Geometry: see drawing. Coordinates: mm, zero at the bounding-box minimum. A direction names the side the tool comes from. Give positions to 0.01 mm unless a question says otherwise; leave off trailing zeros. Write each loop counter-clockwise with the first axis right and the second up, starting at its lowest first coordinate (ties: lowest second). Pieces come first, ordered by that corner, then holes.
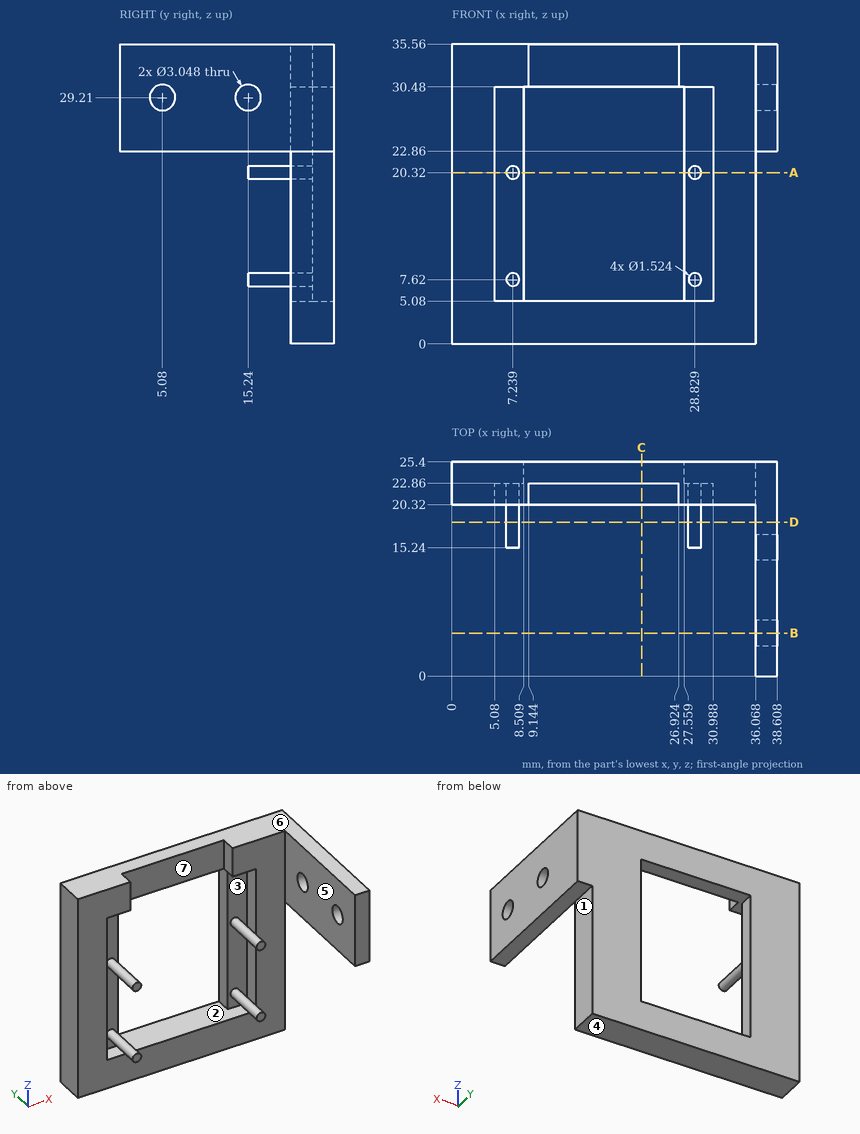
1. Pull-direction query (Z, two-part tool) for the marked faces 1, 2, 3 and 4; classes: pulls with the +Z half, pulls with the -Z half, needs draft (parallel to the pull), parting line crosses it, or undercut.
2. Section query B-B (y = 5.08). Return loops of the section in (x, z), plus the area to 3 significant figures.
3. Line query: probe 1 along Y at (x, z) = (37.65, 29.21); probe 2 along X at (y, z) = (24, 5.5); probe 3 along X at (y, z) = (4, 25.5). Output: solid intervals per line, ascending.
4. Section query C-C (x = 22.5). Return loops of the section in (y, z), plus the area to 3 significant figures.
5. Pin query (flat end, axial travel): P1, Ø4, axis at x = 29, z = 4.5, coming from the -Y side; P2, Ø1.5, axis at y = 23.5, z = 9.5, coming from the +X side; P3, Ø4, axis at y = 15.5, z = 10, coming from the -X side; P4, Ø3, axis at x = 17.5, y = 17, coming from the -Z side. Return the tip coordinate at first contact, or that it passes through.
6. Section query D-D (y = 18.25). Return loops of the section in (x, z), plus the area to 3 significant figures.
7. Access query for the marked faces 5, 6 and 7. Directions: +Z, -Z, +X, -X, +Y, -Y. A direction counts if a zero-diameter tool reaches every point of the face in a straight line with its end or side. Return the directions, or none.
8. Section query A-A (z = 20.32). Return loops of the section in (x, y), plus the area to 3 significant figures.
The answers:
1. face 1: needs draft
1. face 2: undercut
1. face 3: undercut
1. face 4: pulls with the -Z half
2. outline: (36.07, 22.86) - (38.61, 22.86) - (38.61, 27.69) - (36.07, 27.69) - close; (36.07, 30.73) - (38.61, 30.73) - (38.61, 35.56) - (36.07, 35.56) - close
2. area: 24.5 mm2
3. probe 1: y = 0 to 3.56, 6.6 to 13.72, 16.76 to 25.4
3. probe 2: x = 0 to 8.51, 27.56 to 36.07
3. probe 3: x = 36.07 to 38.61
4. outline: (20.32, 0) - (25.4, 0) - (25.4, 5.08) - (20.32, 5.08) - close; (22.86, 30.48) - (25.4, 30.48) - (25.4, 35.56) - (22.86, 35.56) - close
4. area: 38.7 mm2
5. P1: stops at y = 20.32
5. P2: stops at x = 36.07
5. P3: stops at x = 6.58
5. P4: passes through
6. outline: circle Ø1.52 at (7.24, 7.62); circle Ø1.52 at (7.24, 20.32); circle Ø1.52 at (28.83, 7.62); circle Ø1.52 at (28.83, 20.32); (36.07, 22.86) - (38.61, 22.86) - (38.61, 35.56) - (36.07, 35.56) - close
6. area: 39.6 mm2
7. face 5: +Z, -Z, -X, -Y
7. face 6: +Z, +X, -X, +Y, -Y
7. face 7: +Z, -Y
8. outline: (0, 20.32) - (5.08, 20.32) - (5.08, 22.86) - (6.48, 22.86) - (6.48, 15.24) - (8, 15.24) - (8, 22.86) - (8.51, 22.86) - (8.51, 25.4) - (0, 25.4) - close; (27.56, 22.86) - (28.07, 22.86) - (28.07, 15.24) - (29.59, 15.24) - (29.59, 22.86) - (30.99, 22.86) - (30.99, 20.32) - (36.07, 20.32) - (36.07, 25.4) - (27.56, 25.4) - close
8. area: 92.3 mm2
